```python
from build123d import *

# Parameters (mm, degrees)
SKETCH_1_R          = 1.6
EXTRUDE_1_DEPTH     = 2
CUT_EXTRUDE_1_DEPTH = 106.948100502


with BuildPart() as part:
    # Эскиз1 → Бобышка-Вытянуть1 (new body)
    with BuildSketch(Plane(origin=(0, 0, 0), x_dir=(1, 0, 0), z_dir=(0, 1, 0))):
        with BuildLine():
            Line((50, -14), (50, -1.6))
            ThreePointArc((50, -1.6), (48.4, 0), (50, 1.6))
            Line((50, 1.6), (50, 14))
            Line((50, 14), (-50, 14))
            Line((-50, 14), (-54.670248868, 1.785714286))
            ThreePointArc((-54.670248868, 1.785714286), (-55, 0), (-54.670248868, -1.785714286))
            Line((-54.670248868, -1.785714286), (-50, -14))
            Line((-50, -14), (50, -14))
        make_face()
        with Locations(Location((-50, 0, 0), (0, 0, 270))):
            Circle(SKETCH_1_R, mode=Mode.SUBTRACT)
        with Locations(Location((0, 0, 0), (0, 0, 270))):
            Circle(SKETCH_1_R, mode=Mode.SUBTRACT)
    extrude(amount=EXTRUDE_1_DEPTH)

    # Эскиз2 → Вырез-Вытянуть1 (cut, through all)
    with BuildSketch(Plane.ZY.offset(55)):
        Polygon((-14, 0), (-12.645299462, 0), (-13.8, 2), (-14, 2), align=None)
        Polygon((14, 2), (14, 0), (12.645299462, 0), (13.8, 2), align=None)
    extrude(amount=-CUT_EXTRUDE_1_DEPTH, mode=Mode.SUBTRACT)


solid = part.part
```
The model under review builds one solid part; all positions refer to its coordinate system, in mm. Round coordinates to 2 decimals unless told otherwise and drop trailing zeros. Order: outer loops, then holes, each group sorted by start corner. A loop starts at its lowest first (then second) coordinate and runs counter-clockwise, first axis right, second up.
Item 1: Add section C-C, the plane y = 0.65. State the section outline as (x, z) points.
Working result:
outline: (-54.67, -1.79) - (-50.37, -13.02) - (50, -13.02) - (50, -1.6) arc R1.6 cw to (50, 1.6) - (50, 13.02) - (-50.37, 13.02) - (-54.67, 1.79) arc R5 ccw to start; hole circle Ø3.2 at (-50, 0); hole circle Ø3.2 at (0, 0)
Item 2: Add section D-D, the plane x = 26.5. State the section outline as (y, z) points.
Working result:
outline: (0, -12.65) - (2, -13.8) - (2, 13.8) - (0, 12.65) - close
Item 3: Add section A-A, the plane x = 0. State the section outline as (y, z) points.
Working result:
outline: (0, -12.65) - (2, -13.8) - (2, -1.6) - (0, -1.6) - close; (0, 1.6) - (2, 1.6) - (2, 13.8) - (0, 12.65) - close
Item 4: For pin 1 (1 mm diameter, centred on x = 35, y = 1, fed in from +Z), flat-tipped, find the tip position at first contact; note if it passes through.
Working result:
pin 1: stops at z = 13.51
Item 5: To check wall thickness, follow probe 1 along X at (y, z) = (0.5, 0); probe 2 along Z at (x, y) = (-0.5, 1.25); probe 3 along Z at (x, y) = (17, 1.65). State the ranges of each line that lie inside material, in increasing order.
Working result:
probe 1: x = -55 to -51.6, -48.4 to -1.6, 1.6 to 48.4
probe 2: z = -13.37 to -1.52, 1.52 to 13.37
probe 3: z = -13.6 to 13.6
Item 6: Add section B-B, the plane z = 0. State the section outline as (x, y) points, and give its area (3 significant figures).
Working result:
outline: (-55, 0) - (-51.6, 0) - (-51.6, 2) - (-55, 2) - close; (-48.4, 0) - (-1.6, 0) - (-1.6, 2) - (-48.4, 2) - close; (1.6, 0) - (48.4, 0) - (48.4, 2) - (1.6, 2) - close
area: 194 mm2
Item 7: Draft analysis for pull direction Z (two halves, no side actions). For faces 1 (the cylindrical face through (-0.97, 0.99, -1.27)), 2 (the cylindrical face through (-55, 1, 0)), 3 (the flat face through (-52.34, 0.99, -7.88)), state which applies: released by +Z, released by -Z, zero draft, split by the parting line, or undercut.
Working result:
face 1: undercut
face 2: split by the parting line
face 3: released by -Z
